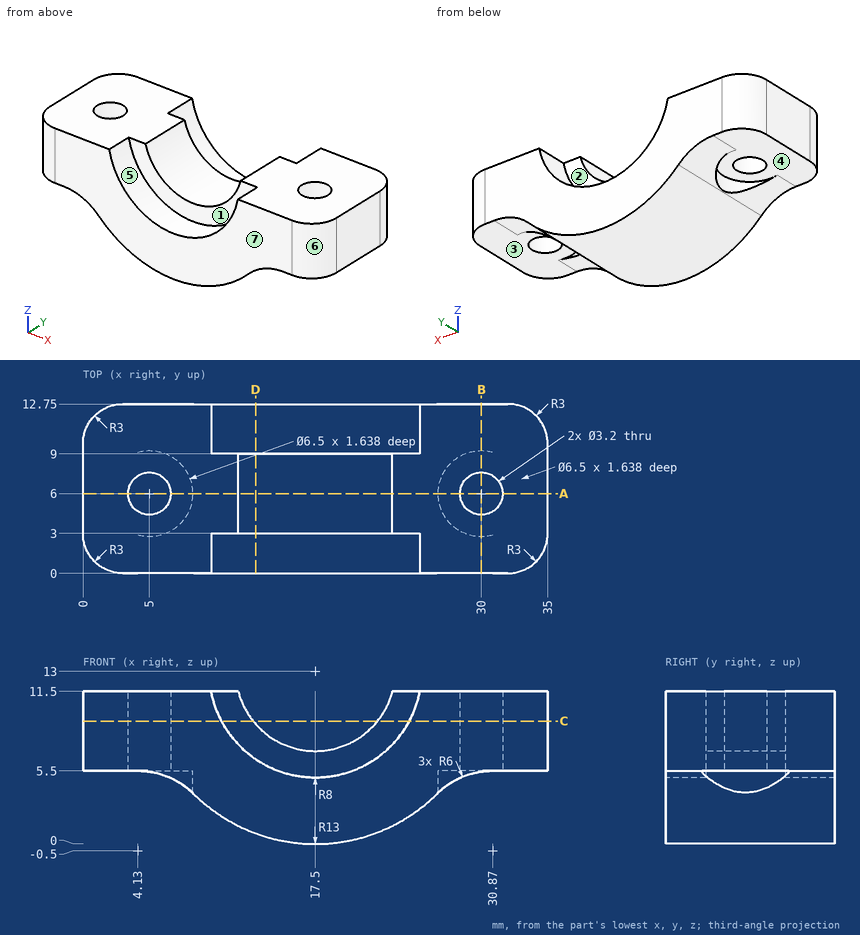
Verification items for this drawing (mm, ordinates from the low corner). A direction names the side the tool comes from. Coordinates: 2 decimals unless noted, no trailing zeros. Order: outer loops, then holes, each group sorted by start corner. A loop starts at its lowest first (then second) coordinate and runs counter-clockwise, first axis right, second up. Notation, with made-up numbers: M 46.25,-25 L 79.25,-25 A9 cw 79.25,-8 Z; hole C 58.25,23 d2. An arc over 180 degrees is marked long. One line per item, written item: value. Start each with the question number.
Item 1: Sectioned sample at D-D on x = 13. Record the cut outline in (y, z).
Item 2: Thickness scan on probe 1 along Y at (x, z) = (5, 7.9); probe 2 along X at (y, z) = (6.5, 8.5); probe 3 along X at (y, z) = (6, 4.9). Record the ranges inside material, lowest first.
Item 3: Depth check by flat-ended pin: P1, Ø2.5, axis at x = 5, y = 6, coming from the -Z side; P2, Ø5, axis at x = 23.5, y = 1.5, coming from the -Z side; P3, Ø6.5, axis at x = 29.5, y = 3.5, coming from the -Z side (1 decimal). Enter the tip coordinate at first touch or a pass-through.
Item 4: Access from +Z, -Z, +X, -X, +Y, -Y to the whole of each face (thin tool, end or side, straight path). Record for the marked faces 1, 2, 3 and 4.
Item 5: Sectioned sample at A-A on y = 6. Record the cut outline in (x, z), then the cut area to 3 significant figures.
Item 6: Sectioned sample at B-B on x = 30. Record the cut outline in (y, z), then the cut area to 3 significant figures.
Item 7: Mould release check, pull along X, two halves, no side actions. Record for the marked faces 5, 6 and 7: pulls with the +X half, pulls with the -X half, needs draft (parallel to the pull), parting line crosses it, or undercut.
Item 8: Sectioned sample at C-C on z = 9.25. Record the cut outline in (x, y), then the cut area to 3 significant figures.
Calculated:
1. outline: M 0,0.8 L 12.75,0.8 L 12.75,6.39 L 9,6.39 L 9,9.03 L 3,9.03 L 3,6.39 L 0,6.39 Z
2. probe 1: 0 to 4.4, 7.6 to 12.75
2. probe 2: 0 to 3.48, 6.52 to 13.53, 21.47 to 28.48, 31.52 to 35
2. probe 3: 8.25 to 26.75
3. P1: through
3. P2: z = 0.48
3. P3: z = 3.4
4. face 1: +Z, -Y
4. face 2: +Z, +Y
4. face 3: -Z, +X
4. face 4: -Z, -X
5. outline: M 0,5.5 L 3.4,5.5 L 3.4,11.5 L 0,11.5 Z; M 6.6,5.5 L 8.25,5.5 L 8.25,3.86 A6 cw 8.35,3.76 A13 ccw 26.65,3.76 A6 cw 26.75,3.86 L 26.75,5.5 L 28.4,5.5 L 28.4,11.5 L 23.31,11.5 A6 cw 11.69,11.5 L 6.6,11.5 Z; M 31.6,5.5 L 35,5.5 L 35,11.5 L 31.6,11.5 Z
5. area: 212 mm^2
6. outline: M 0,5.44 L 2.75,5.44 L 2.75,5.5 L 4.4,5.5 L 4.4,11.5 L 0,11.5 Z; M 7.6,5.5 L 9.25,5.5 L 9.25,5.44 L 12.75,5.44 L 12.75,11.5 L 7.6,11.5 Z
6. area: 57.7 mm^2
7. face 5: undercut
7. face 6: pulls with the +X half
7. face 7: needs draft
8. outline: M 0,3 A3 ccw 3,0 L 10.43,0 L 10.43,3 L 12.82,3 L 12.82,9 L 10.43,9 L 10.43,12.75 L 3,12.75 A3 ccw 0,9.75 Z; M 22.18,3 L 24.57,3 L 24.57,0 L 32,0 A3 ccw 35,3 L 35,9.75 A3 ccw 32,12.75 L 24.57,12.75 L 24.57,9 L 22.18,9 Z; hole C 5,6 d3.2; hole C 30,6 d3.2
8. area: 271 mm^2
